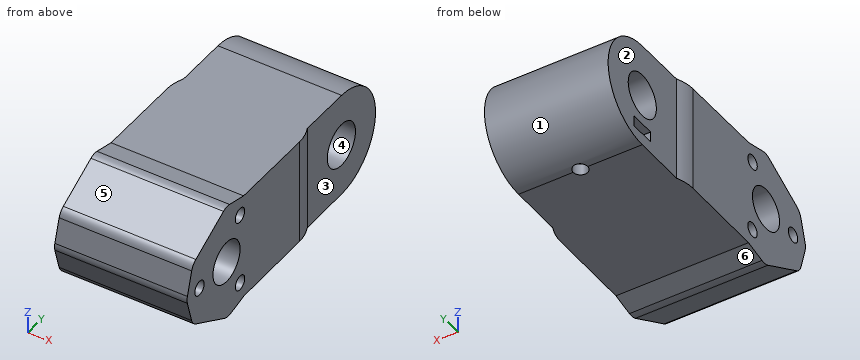
```python
from build123d import *

# Parameters (mm, degrees)
SKETCH3_R                = 4.764999999999999
SKETCH3_R_2              = 1.6499999999999995
SKETCH3_R_3              = 1.6500000000000001
SKETCH3_R_4              = 4.949999999999999
BOSS_EXTRUDE1_DEPTH      = 15
CUT_EXTRUDE2_START       = -13.584871855
CUT_EXTRUDE2_DEPTH       = 26.96953595
CUT_EXTRUDE2_START_2     = -9.35
CUT_EXTRUDE2_2_DEPTH     = 2.4
CUT_EXTRUDE2_START_3     = -12.112585404
CUT_EXTRUDE2_3_OUTLINE_R = 1.65
CUT_EXTRUDE2_3_DEPTH     = 7.445675888


with BuildPart() as part:
    # Sketch3 → Boss-Extrude1 (new, symmetric)
    with BuildSketch(Plane(origin=(0, 0, 0), x_dir=(0, 0, -1), z_dir=(1, 0, 0))):
        with BuildLine():
            Line((0.8367219106320328, 14.181702950289672), (6.032844785264023, 15.69082448784832))
            ThreePointArc((6.032844785264023, 15.69082448784832), (7.085502436432338, 16.24148999245743), (7.8418800486349785, 17.15757597984521))
            Line((7.8418800486349785, 17.15757597984521), (13.230629028910363, 27.2391027259585))
            ThreePointArc((13.230629028910363, 27.2391027259585), (13.56149316864207, 28.279506504021278), (13.498149754436925, 29.369414166277377))
            Line((13.498149754436925, 29.369414166277377), (12.335634292704244, 34.09876588260545))
            Line((12.335634292704244, 34.09876588260545), (12, 69.874079866702))
            ThreePointArc((12, 69.874079866702), (0.03578997764799362, 81.87402649481248), (-11.999786512916659, 69.94565950363487))
            Line((-11.999786512916659, 69.94565950363487), (-12.080609434266979, 33.95094660386098))
            Line((-12.080609434266979, 33.95094660386098), (-13.298066935132345, 28.994347536270237))
            ThreePointArc((-13.298066935132345, 28.994347536270237), (-13.361252777703697, 27.904688590043286), (-13.030421269406453, 26.864544569769336))
            Line((-13.030421269406453, 26.864544569769336), (-7.841880048634967, 17.157575979845202))
            ThreePointArc((-7.841880048634967, 17.157575979845202), (-7.085502436432326, 16.24148999245743), (-6.032844785264015, 15.690824487848316))
            Line((-6.032844785264015, 15.690824487848316), (-0.8367219106320335, 14.18170295028967))
            ThreePointArc((-0.8367219106320335, 14.18170295028967), (1.8e-16, 14.062657036051588), (0.8367219106320328, 14.181702950289672))
        make_face()
        with Locations((1.16e-15, 27.94265703605159)):
            Circle(SKETCH3_R, mode=Mode.SUBTRACT)
        with Locations((0, 18.43265703605159)):
            Circle(SKETCH3_R_2, mode=Mode.SUBTRACT)
        with Locations((8.23590158999005, 32.69765703605151)):
            Circle(SKETCH3_R_3, mode=Mode.SUBTRACT)
        with Locations((-8.19852155344579, 32.659777731318925)):
            Circle(SKETCH3_R_3, mode=Mode.SUBTRACT)
        with Locations((0, 69.874079866702)):
            Circle(SKETCH3_R_4, mode=Mode.SUBTRACT)
    extrude(amount=BOSS_EXTRUDE1_DEPTH, both=True)

    # Cut-Extrude2: read off the stored shape, not the designer's step
    # Cut-Extrude2 outline → Cut-Extrude2 (cut)
    with BuildSketch(Plane.XY.offset(CUT_EXTRUDE2_START)):
        with BuildLine():
            ThreePointArc((-15, 53.515180923), (-14.746794345, 55.751248901), (-14, 57.874079867))
            Line((-14, 57.874079867), (-14, 83))
            Line((-14, 83), (-15, 83))
            Line((-15, 83), (-15, 53.515180923))
        make_face()
        with BuildLine():
            Line((15, 83), (14, 83))
            Line((14, 83), (14, 57.873583349))
            ThreePointArc((14, 57.873583349), (14.746794345, 55.750752383), (15, 53.514684405))
            Line((15, 53.514684405), (15, 83))
        make_face()
    extrude(amount=CUT_EXTRUDE2_DEPTH, mode=Mode.SUBTRACT)

    # Cut-Extrude2 2 outline → Cut-Extrude2 2 (cut)
    with BuildSketch(Plane.XY.offset(CUT_EXTRUDE2_START_2)):
        Polygon((-14, 66.924079867), (1.703183294, 66.924079867), (3.406366588, 69.874079867), (1.703183294, 72.824079867), (-14, 72.824079867), align=None)
    extrude(amount=CUT_EXTRUDE2_2_DEPTH, mode=Mode.SUBTRACT)

    # Cut-Extrude2 3 outline → Cut-Extrude2 3 (cut)
    with BuildSketch(Plane.XY.offset(CUT_EXTRUDE2_START_3)):
        with Locations((0, 69.874079867)):
            Circle(CUT_EXTRUDE2_3_OUTLINE_R)
    extrude(amount=CUT_EXTRUDE2_3_DEPTH, mode=Mode.SUBTRACT)


solid = part.part
```
Read the model definition and answer for the solid it produces. Units are mm, in the model's axes. Face numbers are marked on the shaded views. A direction names the side the tool comes from. Coordinates: 2 decimals unless noted, no trailing zeros. Order: outer loops, then holes, each group sorted by start corner. A loop starts at its lowest first (then second) coordinate and runs counter-clockwise, first axis right, second up. Notation, with made-up numbers: (-16, -28.75) - (29, -28.75) arc R22 cw to (29, 0.25) - close; hole circle Ø7 at (-34.5, 61). An arc over 180 degrees is marked (long way). Answer as a JSON object with one key per item and string values. Group by question number.
Item 1: The mould has two halves that part along Z. Classify the marked faces 4, 5 and 6: +Z half, -Z half, draft (parallel to the pull), parting line (faces both ways), or undercut.
Item 2: Section A-A (z = 0) is taken. Give the vertices of the cut face in (x, y).
Item 3: A tool of negligible diameter and unlimited length cuts with its end or side. For the marked faces 1, 2 and 3, from which of +Z, -Z, +X, -X, +Y, -Y can it reach the whole face along a straight path? Write none if from no direction.
Item 4: Section D-D (x = 8.25) is taken. Give the vertices of the cut face in (y, z) (3 decimals), plus the area to 3 significant figures.
Item 5: Section B-B (y = 25) is taken. Give the vertices of the cut face in (x, z), plus the area to 3 significant figures.
Item 6: Flat-ended cylindrical pins translate along their axes: P1, Ø2, axis at y = 63, z = 1.5, coming from the +X side; P2, Ø4.5, axis at x = 0, y = 69.87, coming from the -Z side; P3, Ø8, axis at x = -7, y = 25.5, coming from the +Z side; P4, Ø4.5, axis at x = -2, y = 70, coming from the +Z side. Find the tip coordinate at first contact, or state that the pin passes through.
Item 7: Consider probe 1 along Y at (x, z) = (-3.75, 0); probe 2 along Y at (x, z) = (-7, -3); probe 3 along Y at (x, z) = (2, -2). Determine where each line is inside the solid, lowest interval first. Write a range as from..to.
Item 8: Section C-C (z = 8.75) is taken. Give the vertices of the cut face in (x, y), plus the area to 3 significant figures.
Results are:
{
 "1": {"face 4": "undercut", "face 5": "+Z half", "face 6": "-Z half"},
 "2": {"outline": "(-15, 14.06) - (15, 14.06) - (15, 16.78) - (-15, 16.78) - close; (-15, 20.08) - (15, 20.08) - (15, 23.18) - (-15, 23.18) - close; (-15, 32.71) - (15, 32.71) - (15, 53.51) arc R10 ccw to (14, 57.87) - (14, 64.92) - (-14, 64.92) - (-14, 57.87) arc R10 ccw to (-15, 53.52) - close; (-14, 74.82) - (14, 74.82) - (14, 81.87) - (-14, 81.87) - close"},
 "3": {"face 1": "+X, -X, +Y", "face 2": "+Z, -Z, -X, +Y", "face 3": "+Z, -Z, +X, +Y"},
 "4": {"outline": "(14.182, -0.837) - (15.691, -6.033) arc R3 ccw to (17.158, -7.842) - (27.239, -13.231) arc R3 ccw to (29.369, -13.498) - (34.099, -12.336) - (69.874, -12) arc R12 ccw to (69.946, 12) - (33.951, 12.081) - (28.994, 13.298) arc R3 ccw to (26.865, 13.03) - (17.158, 7.842) arc R3 ccw to (15.691, 6.033) - (14.182, 0.837) arc R3 ccw to start; hole circle Ø3.3 at (18.433, 0); hole circle Ø9.53 at (27.943, 0); hole circle Ø3.3 at (32.66, 8.199); hole circle Ø3.3 at (32.698, -8.236); hole circle Ø9.9 at (69.874, 0)", "area": "1,340 mm^2"},
 "5": {"outline": "(-15, -12.03) - (15, -12.03) - (15, -3.75) - (-15, -3.75) - close; (-15, 3.75) - (15, 3.75) - (15, 12.03) - (-15, 12.03) - close", "area": "497 mm^2"},
 "6": {"P1": "stops at x = 14", "P2": "stops at z = -12.02", "P3": "stops at z = 13.38", "P4": "stops at z = 12"},
 "7": {"probe 1": "y = 14.06..16.78, 20.08..23.18, 32.71..64.92, 74.82..81.87", "probe 2": "y = 14.81..24.24, 31.64..65.94, 73.81..81.49", "probe 3": "y = 14.52..23.62, 32.27..65.35, 74.4..81.71"},
 "8": {"outline": "(-15, 18.86) - (15, 18.86) - (15, 31.1) - (-15, 31.1) - close; (-15, 34.21) - (15, 34.21) - (15, 53.51) arc R10 ccw to (14, 57.87) - (14, 78.09) - (-14, 78.09) - (-14, 57.87) arc R10 ccw to (-15, 53.52) - close", "area": "1,640 mm^2"}
}
